```python
from build123d import *

# Parameters (mm, degrees)
SKETCH_1_W      = 80
SKETCH_1_H      = 50
SKETCH_1_W_2    = 75
SKETCH_1_H_2    = 45
SKETCH_1_W_3    = 70
SKETCH_1_H_3    = 40
EXTRUDE_1_DEPTH = 2
SKETCH_2_W      = 80
SKETCH_2_H      = 50
SKETCH_2_W_2    = 75
SKETCH_2_H_2    = 45
EXTRUDE_2_DEPTH = 1
SKETCH_3_W      = 75
SKETCH_3_H      = 45
SKETCH_3_W_2    = 70
SKETCH_3_H_2    = 40
EXTRUDE_3_DEPTH = 1


with BuildPart() as part:
    # 스케치1 → 보스-돌출1 (new body)
    # profile 1 of 2: a face of its own
    with BuildSketch(Plane.XY):
        with Locations((-40, 25)):
            Rectangle(SKETCH_1_W, SKETCH_1_H)
        with Locations((-40, 25)):
            Rectangle(SKETCH_1_W_2, SKETCH_1_H_2, mode=Mode.SUBTRACT)
    # profile 2 of 2: a face of its own
    with BuildSketch(Plane.XY):
        with Locations((-40, 25)):
            Rectangle(SKETCH_1_W_2, SKETCH_1_H_2)
        with Locations((-40, 25)):
            Rectangle(SKETCH_1_W_3, SKETCH_1_H_3, mode=Mode.SUBTRACT)
    extrude(amount=EXTRUDE_1_DEPTH)

    # 스케치2 → 보스-돌출2 (add)
    with BuildSketch(Plane.XY.offset(2)):
        with Locations((-40, 25)):
            Rectangle(SKETCH_2_W, SKETCH_2_H)
        with Locations((-40, 25)):
            Rectangle(SKETCH_2_W_2, SKETCH_2_H_2, mode=Mode.SUBTRACT)
    extrude(amount=EXTRUDE_2_DEPTH)

    # 스케치3 → 보스-돌출3 (add)
    with BuildSketch(Plane(origin=(0, 0, 0), x_dir=(-1, 0, 0), z_dir=(0, 0, -1))):
        with Locations((40, 25)):
            Rectangle(SKETCH_3_W, SKETCH_3_H)
        with Locations((40, 25)):
            Rectangle(SKETCH_3_W_2, SKETCH_3_H_2, mode=Mode.SUBTRACT)
    extrude(amount=EXTRUDE_3_DEPTH)


solid = part.part
```
For this review, take the finished solid that the model builds, in its own axes (mm). A direction names the side the tool comes from. Round coordinates to 2 decimals unless told otherwise and drop trailing zeros. Write each loop counter-clockwise with the first axis right and the second up, starting at its lowest first coordinate (ties: lowest second). Pieces come first, ordered by that corner, then holes. Notation, with made-up numbers: (23.5, 15.25) -> (49.5, 15.25) arc R12 cw to (49.5, 32.25) -> close; hole circle Ø10 at (3, 3). An arc over 180 degrees is marked (long way). One line per question, with ' | ' between items. Start each with the question number.
1) Machinability: for faces 1 (the flat face through (-40, 5, 1)), 2 (the flat face through (0, 25, 1)), which of the approach directions +Z, -Z, +X, -X, +Y, -Y give a long, thin tool a straight path to every point of the face, cutting with its end or side? Answer none if there is none.
2) Add section B-B (x = -34). Write out the cut boundary in (y, z), and give its area (3 significant figures).
3) Mouldability with a two-part tool opening along Y and no side actions: class faces 3 (the flat face through (-43, 1, 0)), 4 (the flat face through (-41, 50, 1)), 5 (the flat face through (-5, 25, 1)) as +Y half, -Y half, draft (parallel to the pull), parting line (faces both ways), or undercut.
4) Add section A-A (y = 10.5). Write out the cut boundary in (x, z), and give its area (3 significant figures).
5) For pin 1 Ø0.5 at (x, z) = (-30.5, -0.5) entering from +Y; pin 2 Ø0.5 at (y, z) = (31, -0.5) entering from -X; pin 3 Ø13.5 at (x, y) = (-57, 17.5) entering from +Z, all flat-tipped, find the tip position at first contact; note any pin that passes through.
6) Add section C-C (z = 1.2). Write out the cut boundary in (x, y).
7) Wall thickness on line 1 along Y through (x, z) = (-15, -0.25); line 2 along Y through (x, z) = (-69, 1.75); line 3 along X through (y, z) = (20, -0.3): over which ranges is each line inside the solid? List them lowest first.
Reported:
1) face 1: +Z, -Z | face 2: +Z, -Z, +X, +Y, -Y
2) outline: (0, 0) -> (2.5, 0) -> (2.5, -1) -> (5, -1) -> (5, 2) -> (2.5, 2) -> (2.5, 3) -> (0, 3) -> close; (45, -1) -> (47.5, -1) -> (47.5, 0) -> (50, 0) -> (50, 3) -> (47.5, 3) -> (47.5, 2) -> (45, 2) -> close | area: 30.0 mm²
3) face 3: draft | face 4: +Y half | face 5: undercut
4) outline: (-80, 0) -> (-77.5, 0) -> (-77.5, -1) -> (-75, -1) -> (-75, 2) -> (-77.5, 2) -> (-77.5, 3) -> (-80, 3) -> close; (-5, -1) -> (-2.5, -1) -> (-2.5, 0) -> (0, 0) -> (0, 3) -> (-2.5, 3) -> (-2.5, 2) -> (-5, 2) -> close | area: 30.0 mm²
5) pin 1: stops at y = 47.5 | pin 2: stops at x = -77.5 | pin 3: passes through
6) outline: (-80, 0) -> (0, 0) -> (0, 50) -> (-80, 50) -> close; hole (-75, 5) -> (-5, 5) -> (-5, 45) -> (-75, 45) -> close
7) line 1: y = 2.5 to 5, 45 to 47.5 | line 2: y = 0 to 5, 45 to 50 | line 3: x = -77.5 to -75, -5 to -2.5
